Geometry: final body of the model. Coordinates: model frame, mm. A direction names the side the tool comes from. Round coordinates to 2 decimals unless told otherwise and drop trailing zeros. Loops run counter-clockwise (first coordinate to the right, second up) from the corner with the lowest first, then second, coordinate; pieces in that order, holes last. Notation, with made-up numbers: (57.25, 57) - (90.25, 57) arc R10 cw to (90.25, 70) - close; hole circle Ø11 at (85.5, 71). An arc over 180 degrees is marked (long way). Answer in a Markdown table with one row per item. Add a question column.
from build123d import *

# Parameters (mm, degrees)
SKETCH1_R                  = 59
EXTRUDE1_DEPTH             = 3
EXTRUDE2_DEPTH             = 3
CIRPATTERN1_COUNT          = 13
F_2_5_2_5_DIAMETER_HOLE1_D = 2.5
F_3_0_3_DIAMETER_HOLE1_D   = 3


with BuildPart() as part:
    # Sketch1 → Extrude1 (new, symmetric)
    with BuildSketch(Plane(origin=(0, 0, 0), x_dir=(0, 0, -1), z_dir=(1, 0, 0))):
        Circle(SKETCH1_R)
        Polygon((14.462624243, 25.05), (-14.462624243, 25.05), (-28.925248486, 0), (-14.462624243, -25.05), (14.462624243, -25.05), (28.925248486, 0), align=None, mode=Mode.SUBTRACT)
    extrude(amount=EXTRUDE1_DEPTH, both=True)

    # Sketch2 → Extrude2 (add, symmetric)
    with BuildSketch(Plane(origin=(0, 0, 0), x_dir=(0, 0, -1), z_dir=(1, 0, 0))):
        with BuildLine():
            Line((-2, 67.961805723), (-0.262709442, 61.478149092))
            ThreePointArc((-0.262709442, 61.478149092), (-0.58620663, 59.77173183), (-2.122608272, 58.961805723))
            ThreePointArc((-2.122608272, 58.961805723), (13.210156106, 57.502102359), (27.642670176, 52.123725745))
            ThreePointArc((27.642670176, 52.123725745), (27.166811562, 52.387250915), (26.700820655, 52.667856348))
            Line((26.700820655, 52.667856348), (5.969647024, 65.669469801))
            ThreePointArc((5.969647024, 65.669469801), (2.146386308, 67.37733487), (-2, 67.961805723))
        make_face()
    extrude2 = extrude(amount=EXTRUDE2_DEPTH, both=True)

    # CirPattern1: Extrude2 ×13 about axis
    cirpattern1_axis = Axis((0, 0, 0), (1, 0, 0))
    for i in range(1, CIRPATTERN1_COUNT):
        add(extrude2.rotate(cirpattern1_axis, i * 360 / CIRPATTERN1_COUNT))

    # Ø2.5 (2.5) Diameter Hole1 (through all)
    with Locations(Plane(origin=(3, 0, 0), x_dir=(0, 0, -1), z_dir=(1, 0, 0))):
        with Locations((-14.462624243, 25.05), (14.462624243, 25.05), (28.925248486, 0), (14.462624243, -25.05), (-14.462624243, -25.05), (-28.925248486, 0)):
            Hole(F_2_5_2_5_DIAMETER_HOLE1_D / 2)

    # Ø3.0 (3) Diameter Hole1 (through all)
    with Locations(Plane(origin=(3, 0, 0), x_dir=(0, 0, -1), z_dir=(1, 0, 0))):
        with Locations((0, 25.05)):
            Hole(F_3_0_3_DIAMETER_HOLE1_D / 2)


solid = part.part
1) Contact query for flat-ended pins moving along their axis: pin 1 Ø1 at (x, z) = (-1, -4.5) entering from +Y; pin 2 Ø3 at (x, z) = (2, -22) entering from -Y; pin 3 Ø3 at (x, z) = (-1.5, -3.5) entering from +Y. Output: stop coordinate, or through.
2) Section A-A, the plane z = 7. Return the cut outline in (x, y), and give its area (3 significant figures).
3) Material intervals for line 1 along Z through (x, y) = (-0.3, -25); line 2 along Y through (x, z) = (-0.55, -15.5); line 3 along Y through (x, z) = (0.9, 14), sorted ascending. Write a range as from..to.
4) Reachability of faces 1 (the flat face through (0, 25.05, -7)), 2 (the flat face through (0.04, 44.94, -41.88)), 3 (the flat face through (0.042, -47.719, -43.803)) from +Z, -Z, +X, -X, +Y, -Y: full face, straight path, thin tool, end or side. Return the list, or none.
5) Section B-B, the plane y = -12.5. Return the cut outline in (x, z).
6) Pull-direction query (Y, two-part tool) for faces 4 (the flat face through (-3, -17, 27)), 5 (the cylindrical face through (0.04, 60.67, 29.35)), 6 (the flat face through (0.04, -36.16, -49.66)); classes: pulls with the +Y half, pulls with the -Y half, needs draft (parallel to the pull), parting line crosses it, or undercut.
Evaluation:
| question | item | result |
|---|---|---|
| 1 | pin 1 | stops at y = 66.71 |
| 1 | pin 2 | stops at y = -56.2 |
| 1 | pin 3 | stops at y = 67.42 |
| 2 | outline | (-3, -59.61) - (3, -59.61) - (3, -25.05) - (-3, -25.05) - close; (-3, 25.05) - (3, 25.05) - (3, 59.52) - (-3, 59.52) - close |
| 2 | area | 414 mm² |
| 3 | line 1 | z = -62.86..-15.71, 15.71..53.95, 61.49..63.17 |
| 3 | line 2 | y = -65.92..-60.6, -57.08..-25.75, -24.35..-23.25, 23.25..24.35, 25.75..59.69 |
| 3 | line 3 | y = -58.44..-26.21, 26.21..60.06 |
| 4 | face 1 | +X, -X |
| 4 | face 2 | +X, -X, +Y |
| 4 | face 3 | -Z, +X, -X |
| 5 | outline | (-3, -59.1) - (3, -59.1) - (3, -21.71) - (-3, -21.71) - close; (-3, 21.71) - (3, 21.71) - (3, 62.48) - (-3, 62.48) - close |
| 6 | face 4 | needs draft |
| 6 | face 5 | pulls with the +Y half |
| 6 | face 6 | undercut |
